from build123d import *

# Parameters (mm, degrees)
F1_DEPTH = 76.2
F2_DEPTH = 76.2
F3_R     = 12.7
F4_DEPTH = 76.201
F6_DEPTH = 25.4
F7_R     = 38.1
F8_R     = 19.05
F9_DEPTH = 6.35


with BuildPart() as f1:
    # F0 (on Front) → F1 (new body)
    with BuildSketch(Plane.XZ):
        Polygon((-76.2, 0), (0, 0), (0, 152.4), (-22.206856, 152.4), (-22.206856, 21.336), (-76.2, 21.336), align=None)
    extrude(amount=-F1_DEPTH)

    # F1_face (on face) → F2 (join)
    with BuildSketch(Plane(origin=(-20.778911, 0, 59.558169), x_dir=(1, 0, 0), z_dir=(0, -1, 0))):
        Polygon((-1.427945, -38.222169), (-55.421089, -38.222169), (-55.421089, -59.558169), (20.778911, -59.558169), (20.778911, 92.841831), (-1.427945, 92.841831), align=None)
    extrude(amount=F2_DEPTH)

    # F3 (on face) → F4 (cut, through all)
    with BuildSketch(Plane.YZ):
        with Locations((0, 114.3)):
            Circle(F3_R)
    extrude(amount=-F4_DEPTH, mode=Mode.SUBTRACT)

    # F5 (on face) → F6 (cut)
    with BuildSketch(Plane.XY.offset(21.336)):
        with BuildLine():
            Line((-63.5, 12.7), (-76.2, 12.7))
            Line((-76.2, 12.7), (-76.2, -12.7))
            Line((-76.2, -12.7), (-63.5, -12.7))
            ThreePointArc((-63.5, -12.7), (-50.8, 0), (-63.5, 12.7))
        make_face()
    extrude(amount=-F6_DEPTH, mode=Mode.SUBTRACT)

    # F7
    f7_edges = [f1.edges().sort_by_distance(p)[0] for p in [
        (-11.103428, -76.2, 152.4),
        (-11.103428, 76.2, 152.4),
    ]]
    fillet(f7_edges, radius=F7_R)

    # F8 (on face) → F9 (cut)
    with BuildSketch(Plane(origin=(-22.206856, 0, 0), x_dir=(0, -1, 0), z_dir=(-1, 0, 0))):
        with Locations((0, 114.3)):
            Circle(F8_R)
    extrude(amount=-F9_DEPTH, mode=Mode.SUBTRACT)


solid = f1.part
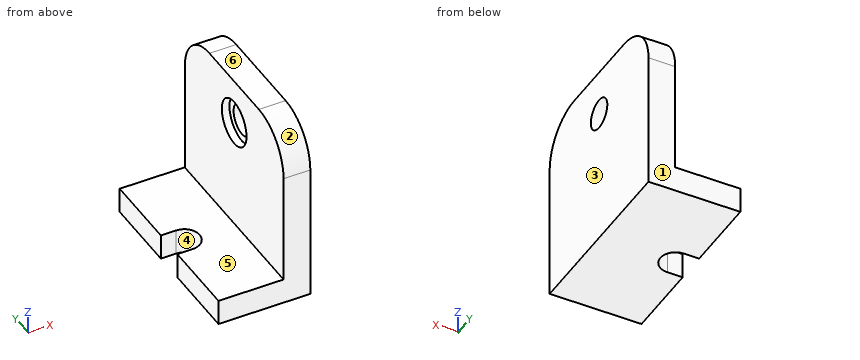
Check sheet for the modelled part. Datum: model origin and axes. Units: mm. Face numbers are marked on the shaded views. A direction names the side the tool comes from. Round coordinates to 2 decimals unless told otherwise and drop trailing zeros. Write each loop counter-clockwise with the first axis right and the second up, starting at its lowest first coordinate (ties: lowest second). Pieces come first, ordered by that corner, then holes. Notation, with made-up numbers: (70, 49) -> (91, 49) arc R22 cw to (91, 86) -> close; hole circle Ø10 at (61, 32.5). An arc over 180 degrees is marked (long way). Answer as CSV lines item,"result". Start each with the question number.
1) Section check C-C on z = 130. Enter the section's corners in (x, y).
2) Section check B-B on x = -9.5. Enter the section's corners in (y, z).
3) Release check for a two-part mould opening along Y. For the marked faces 1, 2, 3 and 4 record: pulls with the +Y half, pulls with the -Y half, needs draft (parallel to the pull), parting line crosses it, or undercut.
4) Go/stop test with flat-tipped pins: P1, Ø19, axis at y = 2.5, z = 110, coming from the -X side; P2, Ø8, axis at y = 58, z = 98.5, coming from the -X side. Record where each tip stops, or that it passes through.
5) Material ranges on line 1 (Z direction, x = -5, y = 0); line 2 (Z direction, x = -19, y = 0); line 3 (Y direction, x = -17, z = 114), recorded low to high. Write a range as from..to.
6) Tool access check on the marked faces 5 and 6. Record the directions out of +Z, -Z, +X, -X, +Y, -Y that give a thin tool (end or side, any length) a straight path to the whole face; none if there is none.
7) Section check A-A on y = 0. Enter the section's corners in (x, z), and give its area (3 significant figures).
8) Section check D-D on z = 112. Enter the section's corners in (x, y), and give its area (3 significant figures).
Found:
1,outline,"(-22.21, -72.81) -> (0, -72.81) -> (0, 72.81) -> (-22.21, 72.81) -> (-22.21, 10.79) -> (-15.86, 10.79) -> (-15.86, -10.79) -> (-22.21, -10.79) -> close"
2,outline,"(-76.2, 0) -> (76.2, 0) -> (76.2, 114.3) arc R38.1 ccw to (38.1, 152.4) -> (-38.1, 152.4) arc R38.1 ccw to (-76.2, 114.3) -> close; hole circle Ø25.4 at (0, 114.3)"
3,face 1,"pulls with the +Y half"
3,face 2,"pulls with the -Y half"
3,face 3,"needs draft"
3,face 4,"undercut"
4,P1,"stops at x = -15.86"
4,P2,"stops at x = -22.21"
5,line 1,"z = 0..101.6, 127..152.4"
5,line 2,"z = 0..95.25, 133.35..152.4"
5,line 3,"y = -76.2..-19.05, 19.05..76.2"
6,face 5,"+Z, -X, +Y, -Y"
6,face 6,"+Z, +X, -X, +Y, -Y"
7,outline,"(-50.8, 0) -> (0, 0) -> (0, 101.6) -> (-15.86, 101.6) -> (-15.86, 95.25) -> (-22.21, 95.25) -> (-22.21, 21.34) -> (-50.8, 21.34) -> close; (-22.21, 133.35) -> (-15.86, 133.35) -> (-15.86, 127) -> (0, 127) -> (0, 152.4) -> (-22.21, 152.4) -> close"
7,area,"3,350 mm^2"
8,outline,"(-22.21, -76.2) -> (0, -76.2) -> (0, -12.49) -> (-15.86, -12.49) -> (-15.86, -18.91) -> (-22.21, -18.91) -> close; (-22.21, 18.91) -> (-15.86, 18.91) -> (-15.86, 12.49) -> (0, 12.49) -> (0, 76.2) -> (-22.21, 76.2) -> close"
8,area,"2,750 mm^2"
